The model under review builds one solid part; all positions refer to its coordinate system, in mm. Round coordinates to 2 decimals unless told otherwise and drop trailing zeros. Write each loop counter-clockwise with the first axis right and the second up, starting at its lowest first coordinate (ties: lowest second). Pieces come first, ordered by that corner, then holes. Notation, with made-up numbers: (41, 80.25) -> (74, 80.25) arc R10 cw to (74, 94.25) -> close; hole circle Ø5 at (-23.5, 85). An arc over 180 degrees is marked (long way). Answer as a JSON object with one key per item and string values. Group by question number.
1) We need section C-C, the plane y = -3. Write out the cut boundary in (x, z).
2) To check wall thickness, follow probe 1 along Y at (x, z) = (39.5, 2.45); probe 2 along Y at (x, z) = (0, 2.2); probe 3 along X at (y, z) = (8, 1.9). State the ranges of each line that lie inside material, in increasing order. Write a range as [from, to].
3) We need section D-D, the plane x = 0. Write out the cut boundary in (y, z).
4) We need section B-B, the plane x = -39.5. Write out the cut boundary in (y, z).
5) Insertion check: pin 1 Ø1 at (y, z) = (-41, 2.5) entering from -X; pin 2 Ø1.5 at (y, z) = (-69, 1.5) entering from -X; pin 3 Ø0.9 at (y, z) = (-9, 2) entering from +X. Each pin has a flat end and moves straight along its axis. Give the tip position at first contact, or say it passes through.
6) We need section A-A, the plane x = -20. Write out the cut boundary in (y, z), then the cut area to 3 significant figures.
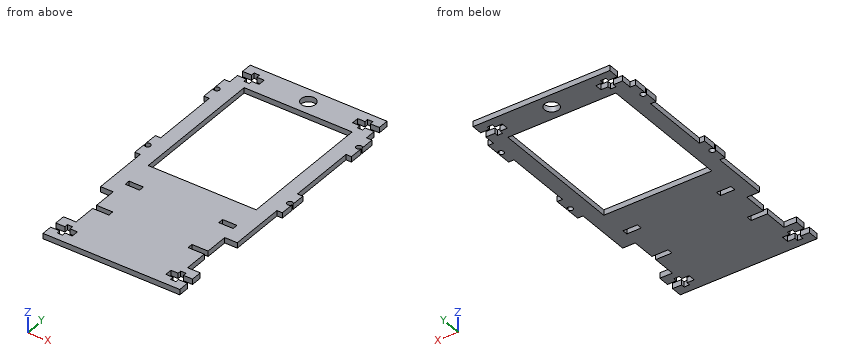
from build123d import *

# Parameters (mm, degrees)
SKETCH_1_W      = 8
SKETCH_1_H      = 3
SKETCH_1_R      = 4
EXTRUDE_1_DEPTH = 3


with BuildPart() as part:
    # 草图1 → 凸台-拉伸1 (new body)
    with BuildSketch(Plane.XY):
        with BuildLine():
            Line((38, 80), (38, 86))
            Line((38, 86), (-38, 86))
            Line((-38, 86), (-38, 80))
            Line((-38, 80), (-33, 80))
            Line((-33, 80), (-33, 82))
            Line((-33, 82), (-30, 82))
            Line((-30, 82), (-30, 80))
            Line((-30, 80), (-26, 80))
            Line((-26, 80), (-26, 76))
            Line((-26, 76), (-30, 76))
            Line((-30, 76), (-30, 74))
            Line((-30, 74), (-33, 74))
            Line((-33, 74), (-33, 76))
            Line((-33, 76), (-38, 76))
            Line((-38, 76), (-38, 70))
            Line((-38, 70), (-41, 70))
            Line((-41, 70), (-41, 62.390512484))
            ThreePointArc((-41, 62.390512484), (-37.95, 62), (-41, 61.609487516))
            Line((-41, 61.609487516), (-41, 54))
            Line((-41, 54), (-38, 54))
            Line((-38, 54), (-38, 16))
            Line((-38, 16), (-41, 16))
            Line((-41, 16), (-41, 8.390512484))
            ThreePointArc((-41, 8.390512484), (-37.95, 8), (-41, 7.609487516))
            Line((-41, 7.609487516), (-41, 0))
            Line((-41, 0), (-38, 0))
            Line((-38, 0), (-38, -31))
            Line((-38, -31), (-31, -31))
            Line((-31, -31), (-31, -44))
            Line((-31, -44), (-22, -44))
            Line((-22, -44), (-22, -47))
            Line((-22, -47), (-31, -47))
            Line((-31, -47), (-31, -60))
            Line((-31, -60), (-38, -60))
            Line((-38, -60), (-38, -66))
            Line((-38, -66), (-33, -66))
            Line((-33, -66), (-33, -64))
            Line((-33, -64), (-30, -64))
            Line((-30, -64), (-30, -66))
            Line((-30, -66), (-26, -66))
            Line((-26, -66), (-26, -70))
            Line((-26, -70), (-30, -70))
            Line((-30, -70), (-30, -72))
            Line((-30, -72), (-33, -72))
            Line((-33, -72), (-33, -70))
            Line((-33, -70), (-38, -70))
            Line((-38, -70), (-38, -76))
            Line((-38, -76), (38, -76))
            Line((38, -76), (38, -70))
            Line((38, -70), (33, -70))
            Line((33, -70), (33, -72))
            Line((33, -72), (30, -72))
            Line((30, -72), (30, -70))
            Line((30, -70), (26, -70))
            Line((26, -70), (26, -66))
            Line((26, -66), (30, -66))
            Line((30, -66), (30, -64))
            Line((30, -64), (33, -64))
            Line((33, -64), (33, -66))
            Line((33, -66), (38, -66))
            Line((38, -66), (38, -60))
            Line((38, -60), (31, -60))
            Line((31, -60), (31, -47))
            Line((31, -47), (22, -47))
            Line((22, -47), (22, -44))
            Line((22, -44), (31, -44))
            Line((31, -44), (31, -31))
            Line((31, -31), (38, -31))
            Line((38, -31), (38, 0))
            Line((38, 0), (41, 0))
            Line((41, 0), (41, 7.609487516))
            ThreePointArc((41, 7.609487516), (37.95, 8), (41, 8.390512484))
            Line((41, 8.390512484), (41, 16))
            Line((41, 16), (38, 16))
            Line((38, 16), (38, 54))
            Line((38, 54), (41, 54))
            Line((41, 54), (41, 61.609487516))
            ThreePointArc((41, 61.609487516), (37.95, 62), (41, 62.390512484))
            Line((41, 62.390512484), (41, 70))
            Line((41, 70), (38, 70))
            Line((38, 70), (38, 76))
            Line((38, 76), (33, 76))
            Line((33, 76), (33, 74))
            Line((33, 74), (30, 74))
            Line((30, 74), (30, 76))
            Line((30, 76), (26, 76))
            Line((26, 76), (26, 80))
            Line((26, 80), (30, 80))
            Line((30, 80), (30, 82))
            Line((30, 82), (33, 82))
            Line((33, 82), (33, 80))
            Line((33, 80), (38, 80))
        make_face()
        with Locations((-26, -21.5)):
            Rectangle(SKETCH_1_W, SKETCH_1_H, mode=Mode.SUBTRACT)
        with Locations((26, -21.5)):
            Rectangle(SKETCH_1_W, SKETCH_1_H, mode=Mode.SUBTRACT)
        Polygon((-30, -5), (-30, 0), (-30, 70), (30, 70), (30, 0), (30, -5), align=None, mode=Mode.SUBTRACT)
        with Locations((0, 78)):
            Circle(SKETCH_1_R, mode=Mode.SUBTRACT)
    extrude(amount=EXTRUDE_1_DEPTH)


solid = part.part
Here are the results:
{
 "1": {"outline": "(-38, 0) -> (-30, 0) -> (-30, 3) -> (-38, 3) -> close; (30, 0) -> (38, 0) -> (38, 3) -> (30, 3) -> close"},
 "2": {"probe 1": "y = [0, 6.45], [9.55, 16], [54, 60.45], [63.55, 70]", "probe 2": "y = [-76, -5], [70, 74], [82, 86]", "probe 3": "x = [-37.95, -30], [30, 37.95]"},
 "3": {"outline": "(-76, 0) -> (-5, 0) -> (-5, 3) -> (-76, 3) -> close; (70, 0) -> (74, 0) -> (74, 3) -> (70, 3) -> close; (82, 0) -> (86, 0) -> (86, 3) -> (82, 3) -> close"},
 "4": {"outline": "(0, 0) -> (6.45, 0) -> (6.45, 3) -> (0, 3) -> close; (9.55, 0) -> (16, 0) -> (16, 3) -> (9.55, 3) -> close; (54, 0) -> (60.45, 0) -> (60.45, 3) -> (54, 3) -> close; (63.55, 0) -> (70, 0) -> (70, 3) -> (63.55, 3) -> close"},
 "5": {"pin 1": "stops at x = -31", "pin 2": "stops at x = -26", "pin 3": "stops at x = 38"},
 "6": {"outline": "(-76, 0) -> (-5, 0) -> (-5, 3) -> (-76, 3) -> close; (70, 0) -> (86, 0) -> (86, 3) -> (70, 3) -> close", "area": "261 mm^2"}
}
